```python
from build123d import *

# Parameters (mm, degrees)
F0_W      = 69.85
F0_H      = 44.45
F1_DEPTH  = 25.4
F2_W      = 44.45
F2_H      = 31.75
F3_DEPTH  = 25.4
F5_DEPTH  = 50.8
F7_DEPTH  = 50.8
F9_DEPTH  = 31.75
F11_DEPTH = 31.75
F13_DEPTH = 25.4
F14_R     = 6.35
F15_DEPTH = 50.8
F17_DEPTH = 25.4


# Not quite as in the source:
# - ends of sketch curves that miss each other by under 0.0002 mm in the source are joined


with BuildPart() as f1:
    # F0 (on Front) → F1 (new body)
    with BuildSketch(Plane.XZ):
        with Locations((34.925, 22.225)):
            Rectangle(F0_W, F0_H)
    extrude(amount=F1_DEPTH)

    # F2 (on face) → F3 (cut)
    with BuildSketch(Plane.XZ.offset(25.4)):
        with Locations((47.625, 28.575)):
            Rectangle(F2_W, F2_H)
    extrude(amount=-F3_DEPTH, mode=Mode.SUBTRACT)

    # F4 (on face) → F5 (cut)
    with BuildSketch(Plane.XY.offset(44.45)):
        with BuildLine():
            ThreePointArc((0, -12.7), (3.7197438789, -3.7197438789), (12.7, 0))
            Line((12.7, 0), (0, 0))
            Line((0, 0), (0, -12.7))
        make_face()
    extrude(amount=-F5_DEPTH, mode=Mode.SUBTRACT)

    # F6 (on face) → F7 (cut)
    with BuildSketch(Plane.XY.offset(44.45)):
        with BuildLine():
            ThreePointArc((12.7, -25.4), (3.7197438789, -21.6802561211), (0, -12.7))
            Line((0, -12.7), (0, -25.4))
            Line((0, -25.4), (12.7, -25.4))
        make_face()
    extrude(amount=-F7_DEPTH, mode=Mode.SUBTRACT)

    # F8 (on face) → F9 (cut)
    with BuildSketch(Plane.XY.offset(44.45)):
        with BuildLine():
            ThreePointArc((25.4, -12.7), (21.6802561211, -21.6802561211), (12.7, -25.4))
            Line((12.7, -25.4), (25.4, -25.4))
            Line((25.4, -25.4), (25.4, -12.7))
        make_face()
    extrude(amount=-F9_DEPTH, mode=Mode.SUBTRACT)

    # F10 (on face) → F11 (cut)
    with BuildSketch(Plane.XY.offset(44.45)):
        with BuildLine():
            ThreePointArc((12.7, 0), (21.6802561211, -3.7197438789), (25.4, -12.7))
            Line((25.4, -12.7), (25.4, 0))
            Line((25.4, 0), (12.7, 0))
        make_face()
    extrude(amount=-F11_DEPTH, mode=Mode.SUBTRACT)

    # F12 (on face) → F13 (cut)
    with BuildSketch(Plane.XY.offset(12.7)):
        with BuildLine():
            ThreePointArc((57.1496006293, -19.0499999874), (50.8, -12.7), (57.1496006293, -6.3500000126))
            Line((57.1496006293, -6.3500000126), (38.3825719247, -6.3562902725))
            ThreePointArc((38.3825719247, -6.3562902725), (42.6889449616, -8.3109130632), (44.45, -12.7))
            ThreePointArc((44.45, -12.7), (42.6333883945, -17.1464468584), (38.2229481372, -19.048809633))
            Line((38.2229481372, -19.048809633), (57.1496006293, -19.0499999874))
        make_face()
        with BuildLine():
            ThreePointArc((57.1496006293, -19.0499999874), (61.6399868594, -17.1902692572), (63.5, -12.7))
            ThreePointArc((63.5, -12.7), (61.6399868594, -8.2097307428), (57.1496006293, -6.3500000126))
            ThreePointArc((57.1496006293, -6.3500000126), (50.8, -12.7), (57.1496006293, -19.0499999874))
        make_face()
        with BuildLine():
            Line((37.81317546, -6.3564811277), (38.3825719247, -6.3562902725))
            ThreePointArc((38.3825719247, -6.3562902725), (38.0978715521, -6.3500003567), (37.81317546, -6.3564811277))
        make_face()
        with BuildLine():
            ThreePointArc((44.45, -12.7), (42.6889449616, -8.3109130632), (38.3825719247, -6.3562902725))
            Line((38.3825719247, -6.3562902725), (37.81317546, -6.3564811277))
            ThreePointArc((37.81317546, -6.3564811277), (31.7505240807, -12.7815815558), (37.9762532721, -19.0487941176))
            Line((37.9762532721, -19.0487941176), (38.2229481372, -19.048809633))
            ThreePointArc((38.2229481372, -19.048809633), (42.6333883945, -17.1464468584), (44.45, -12.7))
        make_face()
        with BuildLine():
            ThreePointArc((37.9762532721, -19.0487941176), (38.0996006293, -19.0499999874), (38.2229481372, -19.048809633))
            Line((38.2229481372, -19.048809633), (37.9762532721, -19.0487941176))
        make_face()
    extrude(amount=-F13_DEPTH, mode=Mode.SUBTRACT)

    # F14 (on face) → F15 (cut)
    with BuildSketch(Plane.XY.offset(44.45)):
        with Locations((12.7, -12.7)):
            Circle(F14_R)
    extrude(amount=-F15_DEPTH, mode=Mode.SUBTRACT)

    # F16 (on face) → F17 (cut)
    with BuildSketch(Plane.XY.offset(12.7)):
        with BuildLine():
            Line((69.85, -25.4), (69.85, -12.7))
            ThreePointArc((69.85, -12.7), (66.1302561211, -21.6802561211), (57.15, -25.4))
            Line((57.15, -25.4), (69.85, -25.4))
        make_face()
        with BuildLine():
            ThreePointArc((57.15, 0), (66.1302561211, -3.7197438789), (69.85, -12.7))
            Line((69.85, -12.7), (69.85, 0))
            Line((69.85, 0), (57.15, 0))
        make_face()
    extrude(amount=-F17_DEPTH, mode=Mode.SUBTRACT)


solid = f1.part
```
Part model, mm, in its own coordinate system. Round coordinates to 2 decimals unless told otherwise and drop trailing zeros. Write each loop counter-clockwise with the first axis right and the second up, starting at its lowest first coordinate (ties: lowest second). Pieces come first, ordered by that corner, then holes. Notation, with made-up numbers: (72, 39.25) -> (85, 39.25) arc R20 ccw to (85, 67.25) -> close; hole circle Ø9 at (18, -5). An arc over 180 degrees is marked (long way). Return JSON: item names as keys, results as strings. Group by question number.
Q1. Saw through at C-C on y = -9.25. Write the cut outline in (x, z), plus the area to 3 significant figures.
Q2. Saw through at B-B on x = 44. Write the cut outline in (y, z), plus the area to 3 significant figures.
Q3. Saw through at D-D on z = 9. Write the cut outline in (x, y).
Q4. Mould opens along Y. For faces 1 (the flat face through (35, -25.4, 6)), 2 (the cylindrical face through (7.66, -16.56, 22.54)), 3 (the flat face through (6.9, -9.7, 44.45)) say: pulls with the +Y half, pulls with the -Y half, needs draft (parallel to the pull), parting line crosses it, or undercut.
Q5. Saw through at A-A on z = 21. Write the cut outline in (x, y).
Q6. Probe L1, parallel to Y at x = 46, z = 4.5; L2, parallel to Z at x = 65, y = -20.5; L3, parallel to Y at x = 17, z = 4. List the from-to ranges inside material, lowest first. Write a range as [from, to].
Q7. Pin check, flat tips, straight feed: pin 1 (1 mm diameter, centred on y = -12, z = 31.5, fed in from +X); pin 2 (12.5 mm diameter, centred on x = 54.5, y = -8.5, fed in from +Z); pin 3 (5 mm diameter, centred on x = 7, z = 23, fed in from -Y). Stop position of each tip, or through.
Answer:
{
 "1": {"outline": "(0.48, 0) -> (7.37, 0) -> (7.37, 44.45) -> (0.48, 44.45) -> close; (18.03, 0) -> (32.77, 0) -> (32.77, 12.7) -> (24.92, 12.7) -> (24.92, 44.45) -> (18.03, 44.45) -> close; (62.48, 0) -> (69.37, 0) -> (69.37, 12.7) -> (62.48, 12.7) -> close", "area": "800 mm2"},
 "2": {"outline": "(-25.4, 0) -> (-19.05, 0) -> (-19.05, 12.7) -> (-25.4, 12.7) -> close; (-6.35, 0) -> (0, 0) -> (0, 12.7) -> (-6.35, 12.7) -> close", "area": "161 mm2"},
 "3": {"outline": "(12.7, -25.4) -> (57.15, -25.4) arc R12.7 ccw to (57.15, 0) -> (12.7, 0) arc R12.7 ccw to start; hole circle Ø12.7 at (12.7, -12.7); hole (38.22, -19.05) -> (57.15, -19.05) arc R6.35 ccw to (57.15, -6.35) -> (38.38, -6.36) arc R6.35 ccw (long way) to start"},
 "4": {"face 1": "pulls with the -Y half", "face 2": "undercut", "face 3": "needs draft"},
 "5": {"outline": "circle Ø25.4 at (12.7, -12.7); hole circle Ø12.7 at (12.7, -12.7)"},
 "6": {"L1": "[-25.4, -19.05], [-6.35, 0]", "L2": "[0, 12.7]", "L3": "[-25.4, -17.37], [-8.03, 0]"},
 "7": {"pin 1": "x = 25.4", "pin 2": "z = 12.7", "pin 3": "y = -24.99"}
}
